Autodesk Inventor part; units mm, degrees
ref_plane "YZ Plane" through (0, 0, 0) normal (1, 0, 0) x (0, 1, 0)
ref_plane "XZ Plane" through (0, 0, 0) normal (0, 1, 0) x (-1, 0, 0)
ref_plane "XY Plane" through (0, 0, 0) normal (0, 0, 1) x (1, 0, 0)
sketch "Sketch23" plane through (0, 0, 0) normal (0, 0, 1) x (1, 0, 0)
  arc A0 (4, 0) -> (0, -4) centre (0, 0) ccw
  line L0 (-4, 0) -> (4, 0)
  line L1 (4, 0) -> (4, -4.25)
  line L2 (0, -4) -> (-3.2578, -4)
  line L3 (-4, -1.4182) -> (-4, 0)
  line L4 (10.5, -4.25) -> (10.5, -7.75)
  line L5 (10.5, -7.75) -> (-4.5, -7.75)
  line L6 (-7.75, -4.25) -> (-7.25, -4.25)
  line L7 (-3.2578, -4) -> (0, -4)
  line L8 (4, -4.25) -> (10.5, -4.25)
  line L9 (-7.25, -4.25) -> (-7.25, -3.75)
  arc A1 (-3.2578, -4) -> (-11.25, -3.75) centre (-7.25, -3.75) ccw
  line L10 (-11.25, -3.75) -> (-11.25, -7.75)
  line L11 (-7.25, -7.75) -> (-11.25, -7.75)
  line L12 (-7.25, -7.75) -> (-4.5, -7.75)
  dimension "d140" = 8
  dimension "d141" = 15
  dimension "d142" = 3.5
  dimension "d143" = 4.25
  dimension "d166" = 0.5
  dimension "d167" = 8
extrude "Extrusion25" add sketch "Sketch23" along normal blind 20 contours L0 A0 | L1 L8 L4 L5 L12 L11 L10 A1 L2 A0 L0
sketch "Sketch30" plane through (0, 0, 20) normal (0, 0, 1) x (1, 0, 0)
  circle A0 centre (0, 0) radius 1.5
  dimension "d168" = 3
extrude "Extrusion30" cut sketch "Sketch30" against normal through all
sketch "Sketch31" plane through (0, 0, 20) normal (0, 0, 1) x (1, 0, 0)
  line L0 (0, -4) -> (10.5, -4)
  line L1 (10.5, -7.75) -> (10.5, -4.25)
  line L2 (10.5, -4) -> (10.5, -7.75)
  line L3 (-11.25, -7.75) -> (10.5, -7.75)
  line L4 (0, -4) -> (10.5, -4)
  line L5 (10.5, -4) -> (10.5, -7.75)
  line L6 (10.5, -7.75) -> (0, -7.75)
  line L7 (0, -7.75) -> (0, -4)
  point P0 (0, 0)
  point P1 (0, -7.75)
extrude "Extrusion31" add sketch "Sketch31" against normal up to surface (20 mm away)
sketch "Sketch32" plane through (0, 0, 20) normal (0, 0, 1) x (1, 0, 0)
  circle A0 centre (0, 0) radius 4
  line L0 (4, -4) -> (10.5, -4)
  line L1 (0, 0) -> (4, 0)
  line L2 (4, 0) -> (4, -4)
  line L3 (4, -4) -> (0, -4)
  line L4 (0, -4) -> (0, 0)
  circle A1 centre (0, 0) radius 1.5
extrude "Extrusion32" cut sketch "Sketch32" against normal blind 5.5 contours L1 A1 L4 A0 | L2 L3 A0 | A0 L4 A1 L1
sketch "Sketch33" plane through (0, 0, 0) normal (0, 0, -1) x (-1, 0, 0)
  circle A0 centre (0, 0) radius 4
  circle A1 centre (0, 0) radius 1.5
  line L0 (-10.5, -4) -> (3.2578, -4)
  line L1 (0, 0) -> (-4, 0)
  line L2 (-4, 0) -> (-4, -4)
  line L3 (-4, -4) -> (0, -4)
  line L4 (0, -4) -> (0, 0)
  point P0 (0, -4)
extrude "Extrusion33" cut sketch "Sketch33" against normal blind 5.5 contours A0 L4 A1 L1 | L1 A1 L4 A0 | A0 L0 L2
fillet "Fillet3" radius 4.25 1 edges at (-3.2578, -4, 10)
sketch "Sketch34" plane through (0, 0, 20) normal (0, 0, 1) x (1, 0, 0)
  arc A0 (-3.7516, -1.8106) -> (-11.25, -3.75) centre (-7.25, -3.75) ccw
  circle A1 centre (-7.25, -3.75) radius 4.1624
  arc A2 (4, 0) -> (0, -4) centre (0, 0) ccw
  line L0 (-11.25, -7.75) -> (10.5, -7.75)
  line L1 (-8.4014, -7.75) -> (-6.0986, -7.75)
  line L2 (-11.25, -3.75) -> (-11.25, -7.75)
  arc A3 (-11.4124, -3.75) -> (-11.25, -7.75) centre (8.552, -4.9427) ccw
  line L3 (-11.25, -7.75) -> (-6.0986, -7.75)
  dimension "d185" = 20
extrude "Extrusion36" add sketch "Sketch34" against normal up to surface (20 mm away) contours L0 L2 A1 | A1 L0 | L2 A3 A1 picked at (-6.2004, -2.965)
sketch "Sketch35" plane through (0, 0, 20) normal (0, 0, 1) x (1, 0, 0)
  line L0 (10.5, -7.75) -> (10.5, -4)
  arc A0 (-11.4124, -3.75) -> (-11.25, -7.75) centre (8.552, -4.9427) ccw
  line L1 (10.5, -7.75) -> (-11.2838, -7.75)
  line L2 (-11.2838, -7.75) -> (-11.2838, -7.5)
  line L3 (-11.2838, -7.5) -> (10.5, -7.5)
  line L4 (10.5, -7.5) -> (10.5, -7.75)
  point P0 (0, 0)
  point P1 (10.5, -7.5)
  point P2 (-11.25, -7.75)
  dimension "d188" = 0.25
extrude "Extrusion37" cut sketch "Sketch35" against normal through all contours L1 A0 L3 L0
sketch "Sketch36" plane through (0, 0, 20) normal (0, 0, 1) x (1, 0, 0)
  line L0 (-11.2838, -7.5) -> (10.5, -7.5)
  line L1 (10.5, -4) -> (-0.0346, -4)
  line L2 (10.5, -7.5) -> (9.5, -7.5)
  line L3 (9.5, -7.5) -> (9.5, -4)
  line L4 (9.5, -4) -> (10.5, -4)
  line L5 (10.5, -4) -> (10.5, -7.5)
  point P0 (0, 0)
  dimension "d191" = 1
extrude "Extrusion38" cut sketch "Sketch36" against normal through all
sketch "Sketch38" plane through (0, 0, 0) normal (0, 0, -1) x (-1, 0, 0)
  arc A0 (11.2838, -7.5) -> (11.4124, -3.75) centre (-8.552, -4.9427) ccw
  line L0 (11.2838, -7.5) -> (10.7838, -6.634)
  line L1 (11.2838, -7.5) -> (12.2838, -7.5) construction
  line L2 (10.7838, -6.634) -> (10.2838, -7.5)
  line L3 (-9.5, -7.5) -> (11.2838, -7.5)
  line L4 (10.2838, -7.5) -> (9.7838, -6.634)
  line L5 (9.7838, -6.634) -> (9.2838, -7.5)
  line L6 (9.2838, -7.5) -> (8.7838, -6.634)
  line L7 (8.7838, -6.634) -> (8.2838, -7.5)
  line L8 (8.2838, -7.5) -> (7.7838, -6.634)
  line L9 (7.7838, -6.634) -> (7.2838, -7.5)
  line L10 (7.2838, -7.5) -> (6.7838, -6.634)
  line L11 (6.7838, -6.634) -> (6.2838, -7.5)
  line L12 (6.2838, -7.5) -> (5.7838, -6.634)
  line L13 (5.7838, -6.634) -> (5.2838, -7.5)
  line L14 (5.2838, -7.5) -> (4.7838, -6.634)
  line L15 (4.7838, -6.634) -> (4.2838, -7.5)
  line L16 (4.2838, -7.5) -> (3.7838, -6.634)
  line L17 (3.7838, -6.634) -> (3.2838, -7.5)
  line L18 (3.2838, -7.5) -> (2.7838, -6.634)
  line L19 (2.7838, -6.634) -> (2.2838, -7.5)
  line L20 (2.2838, -7.5) -> (1.7838, -6.634)
  line L21 (1.7838, -6.634) -> (1.2838, -7.5)
  line L22 (1.2838, -7.5) -> (0.7838, -6.634)
  line L23 (0.7838, -6.634) -> (0.2838, -7.5)
  line L24 (0.2838, -7.5) -> (-0.2162, -6.634)
  line L25 (-0.2162, -6.634) -> (-0.7162, -7.5)
  line L26 (-0.7162, -7.5) -> (-1.2162, -6.634)
  line L27 (-1.2162, -6.634) -> (-1.7162, -7.5)
  line L28 (-1.7162, -7.5) -> (-2.2162, -6.634)
  line L29 (-2.2162, -6.634) -> (-2.7162, -7.5)
  line L30 (-2.7162, -7.5) -> (-3.2162, -6.634)
  line L31 (-3.2162, -6.634) -> (-3.7162, -7.5)
  line L32 (-3.7162, -7.5) -> (-4.2162, -6.634)
  line L33 (-4.2162, -6.634) -> (-4.7162, -7.5)
  line L34 (-4.7162, -7.5) -> (-5.2162, -6.634)
  line L35 (-5.2162, -6.634) -> (-5.7162, -7.5)
  line L36 (-5.7162, -7.5) -> (-6.2162, -6.634)
  line L37 (-6.2162, -6.634) -> (-6.7162, -7.5)
  line L38 (-6.7162, -7.5) -> (-7.2162, -6.634)
  line L39 (-7.2162, -6.634) -> (-7.7162, -7.5)
  line L40 (-7.7162, -7.5) -> (-8.2162, -6.634)
  line L41 (-8.2162, -6.634) -> (-8.7162, -7.5)
  line L42 (11.2838, -7.5) -> (-8.7162, -7.5)
  point P0 (0, 0)
  dimension "d205" = 1
  dimension "d206" = 120
  dimension "d209" = 1
extrude "Extrusion40" cut sketch "Sketch38" against normal through all
sketch "Sketch39" plane through (0, 0, 20) normal (0, 0, 1) x (1, 0, 0)
  arc A0 (-11.4124, -3.75) -> (-11.2838, -7.5) centre (8.552, -4.9427) ccw
  line L0 (-11.4124, -3.75) -> (-11.4124, -7.5)
  line L1 (-10.7838, -6.634) -> (-11.2838, -7.5)
  line L2 (-11.4124, -7.5) -> (-10.7838, -6.634)
  line L3 (-10.7838, -6.634) -> (-11.4124, -3.75)
  point P0 (0, 0)
  point P1 (-11.4124, -6.1353)
  point P2 (-11.3027, -7.3489)
extrude "Extrusion41" add sketch "Sketch39" against normal up to surface (20 mm away) contours L3 L2 A0 L0 | A0 L2 L0
sketch "Sketch40" plane through (0, 0, 20) normal (0, 0, 1) x (1, 0, 0)
  line L0 (-11.4124, -6.1353) -> (-11.4124, -7.5)
  line L1 (-11.4124, -7.5) -> (-11.4124, 0)
  line L2 (-11.4124, -7.5) -> (-3.9124, -7.5) construction
  line L3 (-11.4124, 0) -> (-12.4534, 0)
  line L4 (-12.4534, 0) -> (-12.4534, -7.5)
  line L5 (-12.4534, -7.5) -> (-11.4124, -7.5)
  line L6 (-11.4124, -7.5) -> (-10.7811, -6.63)
  line L7 (-11.4124, -7.5) -> (-10.3375, -7.5) construction
  line L8 (-10.7811, -6.63) -> (-10.7811, -7.5)
  line L9 (-11.4124, -7.5) -> (-10.7811, -7.5)
  point P0 (0, 0)
  dimension "d218" = 90
  dimension "d219" = 54.03
extrude "Extrusion42" cut sketch "Sketch40" against normal through all
sketch "Sketch41" plane through (0, 0, 20) normal (0, 0, 1) x (1, 0, 0)
  line L0 (-11.4124, -7.5) -> (-11.4124, -3.75)
  line L1 (-11.4124, -7.5) -> (-10.2377, -5.8814)
  line L2 (-11.4124, -7.5) -> (-9.4124, -7.5) construction
  line L3 (-9.7838, -6.634) -> (-10.2838, -7.5)
  line L4 (-10.2377, -5.8814) -> (-10.2838, -7.5)
  line L5 (-10.2838, -7.5) -> (-10.7839, -6.6339)
  line L6 (-10.2838, -7.5) -> (-10.7811, -6.6388)
  point P0 (0, 0)
  dimension "d222" = 2
  dimension "d223" = 54.03
extrude "Extrusion43" cut sketch "Sketch41" against normal through all
sketch "Sketch42" plane through (0, 0, 20) normal (0, 0, 1) x (1, 0, 0)
  line L0 (-11.3027, -7.3489) -> (-11.4124, -7.5)
  line L1 (-11.4124, -7.5) -> (-9.6624, -4.4689)
  line L2 (-11.4124, -7.5) -> (-7.9124, -7.5) construction
  line L3 (-9.2838, -7.5) -> (-8.7838, -6.634)
  line L4 (-9.6624, -4.4689) -> (-9.2838, -7.5)
  line L5 (-11.4124, -7.5) -> (-11.4124, -3.75)
  line L6 (-9.2838, -7.5) -> (-11.4124, -7.5)
  arc A0 (-9.6624, -4.4689) -> (-1.2838, -7.5) centre (6.3367, 26.6603) ccw
  line L7 (-9.2838, -7.5) -> (-9.7838, -6.634)
  line L8 (-9.2838, -7.5) -> (-1.2838, -7.5)
  point P0 (0, 0)
  point P1 (-1.2838, -7.5)
  dimension "d226" = 3.5
  dimension "d227" = 60
  dimension "d230" = 35
extrude "Extrusion44" cut sketch "Sketch42" against normal through all
properties part number "Nail"
Here's how the part is built. I have some questions about the finished solid (model axes, mm). A direction names the side the tool comes from. Round coordinates to 2 decimals unless told otherwise and drop trailing zeros. Order: outer loops, then holes, each group sorted by start corner. A loop starts at its lowest first (then second) coordinate and runs counter-clockwise, first axis right, second up. Notation, with made-up numbers: M 44.5,10 L 64.5,10 A23 cw 64.5,38 Z; hole C -34.5,-26 d3. An arc over 180 degrees is marked long. One line per question, with ' | ' between items.
1) I need wall thicknesses on line 1 along X through (y, z) = (0, 9.25); line 2 along X through (y, z) = (-0.5, 11); line 3 along Z through (x, y) = (1, -3.25). Which ranges of each line are inside material? Lowest first, please.
Working result:
line 1: -9.06 to -5.44, -4 to -1.5, 1.5 to 4 | line 2: -9.85 to -4.65, -3.97 to -1.41, 1.41 to 4 | line 3: 5.5 to 14.5
2) I want a section at B-B, the plane y = -5.75. Write out the boundary of the cut face in (x, z).
Working result:
outline: M -11.41,0 L -10.4,0 L -10.4,20 L -11.41,20 Z; M -6.88,0 L 9.5,0 L 9.5,20 L -6.88,20 Z
3) I want a section at C-C, the plane x = -6.5. Write out the boundary of the cut face in (y, z), then the cut area to 3 significant figures.
Working result:
outline: M -5.9,0 L 0.34,0 L 0.34,20 L -5.9,20 Z | area: 125 mm²
4) I want a section at A-A, the plane y = -1.25. Write out the boundary of the cut face in (x, z).
Working result:
outline: M -10.58,0 L -3.92,0 L -3.92,20 L -10.58,20 Z; M -3.8,5.5 L -0.83,5.5 L -0.83,14.5 L -3.8,14.5 Z; M 0.83,5.5 L 4,5.5 L 4,14.5 L 0.83,14.5 Z
5) I want a section at D-D, the plane y = 1.75. Write out the boundary of the cut face in (x, z), then the cut area to 3 significant figures.
Working result:
outline: M -3.6,5.5 L 3.6,5.5 L 3.6,14.5 L -3.6,14.5 Z | area: 64.7 mm²
6) For pin 1 Ø3 at (x, y) = (-4.5, 0.5) entering from -Z; pin 2 Ø5 at (y, z) = (2.5, 16.5) entering from +X; pin 3 Ø6 at (x, z) = (-6, 14.5) entering from -Y; pin 4 Ø1.5 at (x, z) = (-8, 14) entering from -Y, each with a flat end and sliding along its axis, tell me the tip position at first contact or that it passes through.
Working result:
pin 1: z = 0 | pin 2: x = 3.87 | pin 3: y = -7.06 | pin 4: y = -5.59
7) For faces 4 (the face through (0, -2, 14.5)), 5 (the face through (-1.5, 0.07, 10.06)), 6 (the face through (0, -2, 5.5)), which set-ups out of +Z, -Z, +X, -X, +Y, -Y let a thin tool reach every point of the face, with its end or its side?
Working result:
face 4: +Z, +X, +Y | face 5: +Z, -Z | face 6: -Z, +X, +Y
8) If we mould it in two halves opening along X, with no side actions, what happens to faces 1 (the face through (-0.037, -7.073, 9.86)), 2 (the face through (9.5, -6, 10)), 3 (the face through (-3, -4, 20))? For each: +X half, -X half, draft (parallel to the pull), parting line (faces both ways), or undercut.
Working result:
face 1: undercut | face 2: +X half | face 3: draft
